from build123d import *

# Parameters (mm, degrees)
EXTRUDE_1_DEPTH             = 55
EXTRUDE_3_DEPTH             = 2
CUT_EXTRUDE_1_REACH         = 169.242
SKETCH_6_R                  = 3.25
FILLET_1_R                  = 3
SHEET_METAL_1_OUTLINE_W     = 2
SHEET_METAL_1_OUTLINE_H     = 135
SHEET_METAL_1_OUTLINE_W_2   = 23
SHEET_METAL_1_OUTLINE_H_2   = 55
SHEET_METAL_1_DEPTH         = 111
SHEET_START                 = 111
SHEET_METAL_1_2_DEPTH       = 2
SHEET_START_2               = -30
SHEET_METAL_1_3_DEPTH       = 135
SHEET_METAL_1_3_2_DEPTH     = 55
SHEET_METAL_1_3_3_OUTLINE_W = 40
SHEET_METAL_1_3_3_OUTLINE_H = 2
SHEET_METAL_1_3_3_DEPTH     = 135
SHEET_METAL_1_3_4_OUTLINE_W = 20
SHEET_METAL_1_3_4_OUTLINE_H = 2
SHEET_METAL_1_3_4_DEPTH     = 95
SHEET_START_3               = -10
SHEET_METAL_1_3_5_DEPTH     = 10
SHEET_START_4               = -1
SHEET_METAL_1_3_6_DEPTH     = 70


with BuildPart() as part:
    # Sketch 2 → 凸台-拉伸1 (new body)
    with BuildSketch(Plane.XY):
        Polygon((0, 0), (40, 0), (40, 21), (113, 21), (113, 68), (8, 68), (8, 66), (111, 66), (111, 23), (38, 23), (38, 2), (0, 2), align=None)
    extrude(amount=EXTRUDE_1_DEPTH)

    # 草图4 → 凸台-拉伸3 (add)
    with BuildSketch(Plane(origin=(0, 68, 0), x_dir=(1, 0, 0), z_dir=(0, 1, 0))):
        with BuildLine():
            Line((8, 27), (8, 0))
            Line((8, 0), (78, 0))
            ThreePointArc((78, 0), (70.928932188, 2.928932188), (68, 10))
            Line((68, 10), (68, 27))
            ThreePointArc((68, 27), (67.121320344, 29.121320344), (65, 30))
            Line((65, 30), (11, 30))
            ThreePointArc((11, 30), (8.878679656, 29.121320344), (8, 27))
        make_face()
        with BuildLine():
            Line((58, -55), (8, -55))
            Line((8, -55), (8, -102))
            ThreePointArc((8, -102), (8.878679656, -104.121320344), (11, -105))
            Line((11, -105), (45, -105))
            ThreePointArc((45, -105), (47.121320344, -104.121320344), (48, -102))
            Line((48, -102), (48, -65))
            ThreePointArc((48, -65), (50.928932188, -57.928932188), (58, -55))
        make_face()
    extrude(amount=-EXTRUDE_3_DEPTH)

    # 草图6 → 切除-拉伸1 (cut, up to next)
    with BuildSketch(Plane.ZY.offset(-111), mode=Mode.PRIVATE) as cut_extrude_1_sk1:
        with Locations((23, 48)):
            Circle(SKETCH_6_R)
    cut_extrude_1_tool1 = extrude(cut_extrude_1_sk1.sketch, amount=-CUT_EXTRUDE_1_REACH, mode=Mode.PRIVATE) & part.part
    # 草图6 → 切除-拉伸1 (cut, up to next)
    with BuildSketch(Plane.ZY.offset(-111), mode=Mode.PRIVATE) as cut_extrude_1_sk2:
        with Locations((43, 48)):
            Circle(SKETCH_6_R)
    cut_extrude_1_tool2 = extrude(cut_extrude_1_sk2.sketch, amount=-CUT_EXTRUDE_1_REACH, mode=Mode.PRIVATE) & part.part
    add(cut_extrude_1_tool1.solids().sort_by_distance((111, 48, 23))[0], mode=Mode.SUBTRACT)
    add(cut_extrude_1_tool2.solids().sort_by_distance((111, 48, 43))[0], mode=Mode.SUBTRACT)

    # 圆角1
    fillet_1_edges = [part.edges().sort_by_distance(p)[0] for p in [
        (0, 1, 0),
        (0, 1, 55),
    ]]
    fillet(fillet_1_edges, radius=FILLET_1_R)

    # Sheet Metal 1: read off the stored shape, not the designer's step
    # Sheet Metal 1 outline → Sheet Metal 1 (cut)
    with BuildSketch(Plane.YZ):
        with Locations((67, 37.5)):
            Rectangle(SHEET_METAL_1_OUTLINE_W, SHEET_METAL_1_OUTLINE_H)
        with Locations((11.5, 27.5)):
            Rectangle(SHEET_METAL_1_OUTLINE_W_2, SHEET_METAL_1_OUTLINE_H_2)
    extrude(amount=SHEET_METAL_1_DEPTH, mode=Mode.SUBTRACT)

    # Sheet Metal 1 2 outline → Sheet Metal 1 2 (add)
    with BuildSketch(Plane.YZ.offset(SHEET_START)):
        with BuildLine():
            Line((68, 0), (100, 0))
            ThreePointArc((100, 0), (107.071067812, -2.928932188), (110, -10))
            Line((110, -10), (110, -27))
            ThreePointArc((110, -27), (110.878679656, -29.121320344), (113, -30))
            Line((113, -30), (167, -30))
            ThreePointArc((167, -30), (169.121320344, -29.121320344), (170, -27))
            Line((170, -27), (170, 102))
            ThreePointArc((170, 102), (169.121320344, 104.121320344), (167, 105))
            Line((167, 105), (133, 105))
            ThreePointArc((133, 105), (130.878679656, 104.121320344), (130, 102))
            Line((130, 102), (130, 65))
            ThreePointArc((130, 65), (127.071067812, 57.928932188), (120, 55))
            Line((120, 55), (68, 55))
            Line((68, 55), (68, 0))
        make_face()
        with BuildLine():
            Line((21, 0), (21, 55))
            Line((21, 55), (-105, 55))
            ThreePointArc((-105, 55), (-107.121320344, 54.121320344), (-108, 52))
            Line((-108, 52), (-108, 3))
            ThreePointArc((-108, 3), (-107.121320344, 0.878679656), (-105, 0))
            Line((-105, 0), (21, 0))
        make_face()
    extrude(amount=SHEET_METAL_1_2_DEPTH)

    # Sheet Metal 1 3: read off the stored shape, not the designer's step
    # Sheet Metal 1 3 outline → Sheet Metal 1 3 (cut)
    with BuildSketch(Plane.XY.offset(SHEET_START_2)):
        with BuildLine():
            ThreePointArc((113, 24), (112.449489743, 22.267949192), (111, 21.171572875))
            Line((111, 21.171572875), (111, -108))
            Line((111, -108), (113, -108))
            Line((113, -108), (113, 24))
        make_face()
        with BuildLine():
            ThreePointArc((111, 67.828427125), (112.449489743, 66.732050808), (113, 65))
            Line((113, 65), (113, 170))
            Line((113, 170), (111, 170))
            Line((111, 170), (111, 67.828427125))
        make_face()
    extrude(amount=SHEET_METAL_1_3_DEPTH, mode=Mode.SUBTRACT)

    # Sheet Metal 1 3 2 outline → Sheet Metal 1 3 2 (add)
    with BuildSketch(Plane.XY):
        with BuildLine():
            Line((37, 2), (0, 2))
            Line((0, 2), (0, 0))
            Line((0, 0), (37, 0))
            ThreePointArc((37, 0), (39.121320344, 0.878679656), (40, 3))
            Line((40, 3), (40, 20))
            ThreePointArc((40, 20), (40.292893219, 20.707106781), (41, 21))
            Line((41, 21), (110, 21))
            ThreePointArc((110, 21), (110.507305936, 21.043204321), (111, 21.171572875))
            Line((111, 21.171572875), (111, 24))
            ThreePointArc((111, 24), (110.707106781, 23.292893219), (110, 23))
            Line((110, 23), (41, 23))
            ThreePointArc((41, 23), (38.878679656, 22.121320344), (38, 20))
            Line((38, 20), (38, 3))
            ThreePointArc((38, 3), (37.707106781, 2.292893219), (37, 2))
        make_face()
        with BuildLine():
            ThreePointArc((110, 66), (110.707106781, 65.707106781), (111, 65))
            Line((111, 65), (111, 67.828427125))
            ThreePointArc((111, 67.828427125), (110.507305936, 67.956795679), (110, 68))
            Line((110, 68), (8, 68))
            Line((8, 68), (8, 66))
            Line((8, 66), (110, 66))
        make_face()
    extrude(amount=SHEET_METAL_1_3_2_DEPTH)

    # Sheet Metal 1 3 3 outline → Sheet Metal 1 3 3 (add)
    with BuildSketch(Plane.XY.offset(SHEET_START_2)):
        with Locations((28, 67)):
            Rectangle(SHEET_METAL_1_3_3_OUTLINE_W, SHEET_METAL_1_3_3_OUTLINE_H)
    extrude(amount=SHEET_METAL_1_3_3_DEPTH)

    # Sheet Metal 1 3 4 outline → Sheet Metal 1 3 4 (add)
    with BuildSketch(Plane.XY.offset(SHEET_START_2)):
        with Locations((58, 67)):
            Rectangle(SHEET_METAL_1_3_4_OUTLINE_W, SHEET_METAL_1_3_4_OUTLINE_H)
    extrude(amount=SHEET_METAL_1_3_4_DEPTH)

    # Sheet Metal 1 3 5 outline → Sheet Metal 1 3 5 (add)
    with BuildSketch(Plane.XY.offset(SHEET_START_3)):
        with BuildLine():
            Line((68, 68), (68, 66))
            Line((68, 66), (110, 66))
            ThreePointArc((110, 66), (110.707106781, 65.707106781), (111, 65))
            Line((111, 65), (111, 67.828427125))
            ThreePointArc((111, 67.828427125), (110.507305936, 67.956795679), (110, 68))
            Line((110, 68), (68, 68))
        make_face()
    extrude(amount=SHEET_METAL_1_3_5_DEPTH)

    # Sheet Metal 1 3 6 outline → Sheet Metal 1 3 6 (cut)
    with BuildSketch(Plane(origin=(0, 0, 0), x_dir=(1, 0, 0), z_dir=(0, 1, 0)).offset(SHEET_START_4)):
        with BuildLine():
            Line((0, -55), (3, -55))
            ThreePointArc((3, -55), (0.878679656, -54.121320344), (0, -52))
            Line((0, -52), (0, -55))
        make_face()
        with BuildLine():
            Line((0, 0), (0, -3))
            ThreePointArc((0, -3), (0.878679656, -0.878679656), (3, 0))
            Line((3, 0), (0, 0))
        make_face()
        with BuildLine():
            ThreePointArc((11, -105), (8.878679656, -104.121320344), (8, -102))
            Line((8, -102), (8, -105))
            Line((8, -105), (11, -105))
        make_face()
        with BuildLine():
            Line((8, 30), (8, 27))
            ThreePointArc((8, 27), (8.878679656, 29.121320344), (11, 30))
            Line((11, 30), (8, 30))
        make_face()
        with BuildLine():
            ThreePointArc((48, -102), (47.121320344, -104.121320344), (45, -105))
            Line((45, -105), (48, -105))
            Line((48, -105), (48, -102))
        make_face()
        with BuildLine():
            Line((68, 30), (65, 30))
            ThreePointArc((65, 30), (67.121320344, 29.121320344), (68, 27))
            Line((68, 27), (68, 30))
        make_face()
        with BuildLine():
            Line((68, -55), (58, -55))
            ThreePointArc((58, -55), (50.928932188, -57.928932188), (48, -65))
            Line((48, -65), (68, -65))
            Line((68, -65), (68, -55))
        make_face()
        with BuildLine():
            ThreePointArc((68, 10), (70.928932188, 2.928932188), (78, 0))
            Line((78, 0), (111, 0))
            Line((111, 0), (111, 10))
            Line((111, 10), (68, 10))
        make_face()
    extrude(amount=SHEET_METAL_1_3_6_DEPTH, mode=Mode.SUBTRACT)


solid = part.part
The model under review builds one solid part; all positions refer to its coordinate system, in mm. A direction names the side the tool comes from. Round coordinates to 2 decimals unless told otherwise and drop trailing zeros. Order: outer loops, then holes, each group sorted by start corner. A loop starts at its lowest first (then second) coordinate and runs counter-clockwise, first axis right, second up. Notation, with made-up numbers: (8.5, -34) -> (42.5, -34) arc R24 cw to (42.5, -16) -> close; hole circle Ø8 at (35.25, -27). An arc over 180 degrees is marked (long way). Return JSON: item names as keys, results as strings.
1. The part is to be moulded in two halves that separate along Y. For faces 1 (the face through (48, 68, 37)), 2 (the face through (38, 12, 27)), 3 (the face through (67.1, 66.99, -29.14)), say which applies: +Y half, -Y half, draft (parallel to the pull), parting line (faces both ways), or undercut.
Answer block:
{"face 1": "+Y half", "face 2": "undercut", "face 3": "draft"}
2. Insertion check: P1, Ø10.5, axis at y = 48, z = 43, coming from the -X side; P2, Ø8, axis at y = 17.5, z = 49, coming from the +X side; P3, Ø5, axis at y = 14, z = 23, coming from the +X side. Each pin has a flat end and moves straight along its axis. Give the tip position at first contact, or say it passes through.
Answer block:
{"P1": "stops at x = 111", "P2": "stops at x = 111.66", "P3": "stops at x = 40"}
3. Take a section at B-B (y = 48). Write out the cut boundary in (x, z).
Answer block:
{"outline": "(111, 0) -> (113, 0) -> (113, 19.75) -> (111, 19.75) -> close; (111, 26.25) -> (113, 26.25) -> (113, 39.75) -> (111, 39.75) -> close; (111, 46.25) -> (113, 46.25) -> (113, 55) -> (111, 55) -> close"}
4. For L1, parallel to X at y = 35, z = 48; L2, parallel to Y at x = 23, z = 21; L3, parallel to Y at x = 34, z = -5, list the stretches that pass through material, from the lowest coordinate up. Write a range as [from, to].
Answer block:
{"L1": "x = [111, 113]", "L2": "y = [0, 2], [66, 68]", "L3": "y = [66, 68]"}
5. Take a section at C-C (z = 43). Write out the cut boundary in (x, y).
Answer block:
{"outline": "(0, 0) -> (37, 0) arc R3 ccw to (40, 3) -> (40, 20) arc R1 cw to (41, 21) -> (110, 21) arc R3 ccw to (113, 24) -> (113, 44.75) -> (111, 44.75) -> (111, 24) arc R1 cw to (110, 23) -> (41, 23) arc R3 ccw to (38, 20) -> (38, 3) arc R1 cw to (37, 2) -> (0, 2) -> close; (8, 66) -> (110, 66) arc R1 cw to (111, 65) -> (111, 51.25) -> (113, 51.25) -> (113, 65) arc R3 ccw to (110, 68) -> (8, 68) -> close"}
6. Take a section at D-D (z = 10.5). Write out the cut boundary in (x, y), then the cut area to 3 significant figures.
Answer block:
{"outline": "(0, 0) -> (37, 0) arc R3 ccw to (40, 3) -> (40, 20) arc R1 cw to (41, 21) -> (110, 21) arc R3 ccw to (113, 24) -> (113, 65) arc R3 ccw to (110, 68) -> (8, 68) -> (8, 66) -> (110, 66) arc R1 cw to (111, 65) -> (111, 24) arc R1 cw to (110, 23) -> (41, 23) arc R3 ccw to (38, 20) -> (38, 3) arc R1 cw to (37, 2) -> (0, 2) -> close", "area": "557 mm²"}
7. For faces 4 (the face through (47, 66, 37)), 5 (the face through (66, 22, 55)), 6 (the face through (40, 11, 27)), list the 3-axis set-ups (+Z, -Z, +X, -X, +Y, -Y) from which the entire face can be reached by the end or side of a thin tool; tool diameter is ignored.
Answer block:
{"face 4": "+Z, -Z, -X", "face 5": "+Z, +X, -Y", "face 6": "+Z, -Z, +X, -Y"}
8. Take a section at A-A (x = 85). Write out the cut boundary in (y, z).
Answer block:
{"outline": "(21, 0) -> (23, 0) -> (23, 55) -> (21, 55) -> close; (66, 0) -> (68, 0) -> (68, 55) -> (66, 55) -> close"}
